Model file for the job. Use its own axes, mm. Face numbers are marked on the shaded views. A direction names the side the tool comes from. Coordinates: 2 decimals unless noted, no trailing zeros. Write each loop counter-clockwise with the first axis right and the second up, starting at its lowest first coordinate (ties: lowest second). Pieces come first, ordered by that corner, then holes.
Q1. Which spindle directions (+Z, -Z, +X, -X, +Y, -Y) get a long thin tool onto all of the face, cutting with end or side? Do the marked faces 5, 6 and 7. Say none if no direction does.
Q2. Pin check, flat tips, straight feed: P1, Ø1, axis at x = 7.5, z = 0.5, coming from the -Y side; P2, Ø2, axis at x = -2.5, z = -1, coming from the -Y side; P3, Ø8, axis at x = 0, z = 0, coming from the -Y side. Stop position of each tip, or through.
Q3. Band-saw the part on A-A, the plane y = -5. Write the cut outline in (x, z), plus the area to 3 significant figures.
Q4. Pull direction Z, two halves, no side cores. Call the marked faces 1, 2, 3 and 4: released by +Z, released by -Z, zero draft, split by the parting line, or undercut.
Q5. Drill centre lines: probe 1 along Z at (x, y) = (0, -6); probe 2 along Y at (x, z) = (7.5, 0); probe 3 along X at (y, z) = (-12, 1.25). Where is each one in solid material? Low to high.
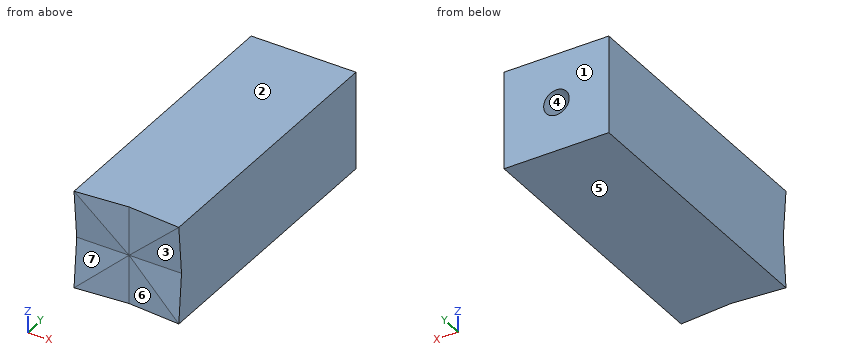
from build123d import *

# Parameters (mm, degrees)
SKETCH1_W             = 20.5
SKETCH1_H             = 19.16
BOSS_EXTRUDE1_DEPTH   = 55.2
CUT_EXTRUDE3_DEPTH    = 60.657911462
CUT_EXTRUDE4_DEPTH    = 60.322913785
M6_TAPPED_HOLE1_D     = 5
M6_TAPPED_HOLE1_DEPTH = 15
M6_TAPPED_HOLE1_TIP   = 1.502151548


with BuildPart() as part:
    # Sketch1 → Boss-Extrude1 (new body)
    with BuildSketch(Plane(origin=(0, 0, 0), x_dir=(1, 0, 0), z_dir=(0, 1, 0))):
        Rectangle(SKETCH1_W, SKETCH1_H)
    extrude(amount=-BOSS_EXTRUDE1_DEPTH)

    # Sketch5 → Cut-Extrude3 (cut, through all)
    with BuildSketch(Plane(origin=(10.25, 0, 0), x_dir=(0, 0, -1), z_dir=(1, 0, 0))):
        Polygon((-9.58, -55.2), (0, -54.361858603), (9.58, -55.2), align=None)
    extrude(amount=-CUT_EXTRUDE3_DEPTH, mode=Mode.SUBTRACT)

    # Sketch6 → Cut-Extrude4 (cut, through all)
    with BuildSketch(Plane(origin=(0, 0, -9.58), x_dir=(-1, 0, 0), z_dir=(0, 0, -1))):
        Polygon((-10.25, -55.2), (0, -54.361858603), (10.25, -55.2), align=None)
    extrude(amount=-CUT_EXTRUDE4_DEPTH, mode=Mode.SUBTRACT)

    # M6 Tapped Hole1
    with Locations(Plane(origin=(0, 0, 0), x_dir=(1, 0, 0), z_dir=(0, 1, 0))):
        with Locations((0, 0)):
            Hole(M6_TAPPED_HOLE1_D / 2, depth=M6_TAPPED_HOLE1_DEPTH)
            with Locations((0, 0, -(M6_TAPPED_HOLE1_DEPTH + M6_TAPPED_HOLE1_TIP / 2))):  # 118° drill point
                Cone(0, M6_TAPPED_HOLE1_D / 2, M6_TAPPED_HOLE1_TIP, mode=Mode.SUBTRACT)


solid = part.part
Answer sheet:
1. face 5: -Z, +X, -X, +Y, -Y
1. face 6: +Z, -Z, -Y
1. face 7: +X, -X, -Y
2. P1: stops at y = -54.45
2. P2: stops at y = -54.54
2. P3: stops at y = -54.6
3. outline: (-10.25, -9.58) - (10.25, -9.58) - (10.25, 9.58) - (-10.25, 9.58) - close; hole circle Ø5 at (0, 0)
3. area: 373 mm2
4. face 1: zero draft
4. face 2: released by +Z
4. face 3: undercut
4. face 4: undercut
5. probe 1: z = -9.58 to -2.5, 2.5 to 9.58
5. probe 2: y = -54.36 to 0
5. probe 3: x = -10.25 to -2.17, 2.17 to 10.25
